from build123d import *

# Parameters (mm, degrees)
P_IDAT_VYSUNUT_M1_DEPTH = 5
ZAOBLIT1_R              = 0.2


with BuildPart() as part:
    # Skica1 → Přidat vysunutím1 (new body)
    with BuildSketch(Plane.XY):
        with BuildLine():
            ThreePointArc((-1.931217233, -4.98), (0, -7.5), (1.931217233, -4.98))
            ThreePointArc((1.931217233, -4.98), (1.950012982, -3.874641932), (2.553134647, -2.948135593))
            ThreePointArc((2.553134647, -2.948135593), (3.850518803, 0.619277763), (1.5, 3.6))
            Line((1.5, 3.6), (1.5, 5.031152949))
            ThreePointArc((1.5, 5.031152949), (5.123560056, 1.145265189), (3.49942144, -3.913636364))
            ThreePointArc((3.49942144, -3.913636364), (3.217064036, -4.343555698), (3.185747809, -4.856951872))
            ThreePointArc((3.185747809, -4.856951872), (0, -8.75), (-3.185747809, -4.856951872))
            ThreePointArc((-3.185747809, -4.856951872), (-3.217064036, -4.343555698), (-3.49942144, -3.913636364))
            ThreePointArc((-3.49942144, -3.913636364), (-5.123560056, 1.145265189), (-1.5, 5.031152949))
            Line((-1.5, 5.031152949), (-1.5, 3.6))
            ThreePointArc((-1.5, 3.6), (-3.850518803, 0.619277763), (-2.553134647, -2.948135593))
            ThreePointArc((-2.553134647, -2.948135593), (-1.950012982, -3.874641932), (-1.931217233, -4.98))
        make_face()
    extrude(amount=P_IDAT_VYSUNUT_M1_DEPTH)

    # Zaoblit1
    zaoblit1_edges = [part.edges().sort_by_distance(p)[0] for p in [
        (1.5, 5.031152949, 2.5),
        (-1.5, 5.031152949, 2.5),
    ]]
    fillet(zaoblit1_edges, radius=ZAOBLIT1_R)


solid = part.part
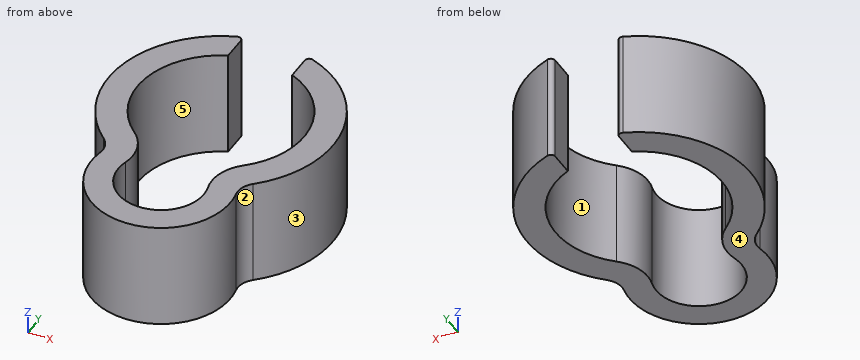
Design review of the part built by this model. Coordinates are the model's own, in mm. Face numbers are marked on the shaded views. A direction names the side the tool comes from. Round coordinates to 2 decimals unless told otherwise and drop trailing zeros. Write each loop counter-clockwise with the first axis right and the second up, starting at its lowest first coordinate (ties: lowest second). Pieces come first, ordered by that corner, then holes. Notation, with made-up numbers: (-3.75, -26) - (5.25, -26) arc R19 cw to (5.25, -2) - close; hole circle Ø8 at (80.25, 39.25). An arc over 180 degrees is marked (long way). Return JSON: item names as keys, results as strings. Group by question number.
Item 1: Machinability: for the marked faces 1 and 2, which of the approach directions +Z, -Z, +X, -X, +Y, -Y give a long, thin tool a straight path to every point of the face, cutting with its end or side? Answer none if there is none.
Item 2: We need section B-B on x = 3.75. Write out the cut boundary in (y, z), and give its area (3 significant figures).
Item 3: For probe 1 along X at (y, z) = (-5.5, 1.85); probe 2 along X at (y, z) = (-4.75, 2.6); probe 3 along Y at (x, z) = (3.5, 3.55), list the stretches that pass through material, from the lowest coordinate up. Write a range as [from, to].
Item 4: Insertion check: P1, Ø3, axis at y = -7, z = 2.5, coming from the -X side; P2, Ø2, axis at y = 1.5, z = 1, coming from the +X side; P3, Ø1, axis at x = 0, z = 3.5, coming from the +Y side. Each pin has a flat end and moves straight along its axis. Give the tip position at first contact, or say it passes through.
Item 5: We need section D-D on z = 1.5. Write out the cut boundary in (x, y), and give its area (3 significant figures).
Item 6: We need section C-C on x = 0. Write out the cut boundary in (y, z).
Item 7: The part is to be moulded in two halves that separate along Y. For the marked faces 3, 4 and 5, say which applies: pulls with the +Y half, pulls with the -Y half, needs draft (parallel to the pull), parting line crosses it, or undercut.
Item 8: We need section A-A on y = -5.5. Write out the cut boundary in (x, z), and give its area (3 significant figures).
Model answer:
{
 "1": {"face 1": "+Z, -Z", "face 2": "+Z, -Z, +X"},
 "2": {"outline": "(-3.67, 0) - (-1.07, 0) - (-1.07, 5) - (-3.67, 5) - close; (1.07, 0) - (3.67, 0) - (3.67, 5) - (1.07, 5) - close", "area": "26.0 mm²"},
 "3": {"probe 1": "x = [-3.25, -2], [2, 3.25]", "probe 2": "x = [-3.17, -1.88], [1.88, 3.17]", "probe 3": "y = [-3.91, -1.72], [1.72, 3.91]"},
 "4": {"P1": "stops at x = -3.25", "P2": "stops at x = 5.23", "P3": "stops at y = -7.44"},
 "5": {"outline": "(-3.5, -3.91) arc R1 cw to (-3.19, -4.86) arc R3.25 ccw (long way) to (3.19, -4.86) arc R1 cw to (3.5, -3.91) arc R5.25 ccw to (1.77, 4.94) arc R0.2 ccw to (1.5, 4.76) - (1.5, 3.6) arc R3.9 cw to (2.55, -2.95) arc R2 ccw to (1.93, -4.98) arc R2 cw (long way) to (-1.93, -4.98) arc R2 ccw to (-2.55, -2.95) arc R3.9 cw to (-1.5, 3.6) - (-1.5, 4.76) arc R0.2 ccw to (-1.77, 4.94) arc R5.25 ccw to start", "area": "41.9 mm²"},
 "6": {"outline": "(-8.75, 0) - (-7.5, 0) - (-7.5, 5) - (-8.75, 5) - close"},
 "7": {"face 3": "parting line crosses it", "face 4": "needs draft", "face 5": "undercut"},
 "8": {"outline": "(-3.25, 0) - (-2, 0) - (-2, 5) - (-3.25, 5) - close; (2, 0) - (3.25, 0) - (3.25, 5) - (2, 5) - close", "area": "12.5 mm²"}
}
